Work out the finished part from the listing and answer in its coordinate system (mm). A direction names the side the tool comes from. Round coordinates to 2 decimals unless told otherwise and drop trailing zeros. Write each loop counter-clockwise with the first axis right and the second up, starting at its lowest first coordinate (ties: lowest second). Pieces come first, ordered by that corner, then holes.
1. Determine the mould class of faces 3 (the face through (1.588, 2, -7)), 4 (the face through (-5.796, 1.565, -7.559)), 5 (the face through (-2, 0, 6.2)) for opening direction X: pulls with the +X half, pulls with the -X half, needs draft (parallel to the pull), parting line crosses it, or undercut.
2. Straight lines are drawn through the part: probe 1 along X at (y, z) = (0.75, 0) (3 decimals); probe 2 along Z at (x, y) = (-5, 0.85); probe 3 along X at (y, z) = (2.4, -3.5). For each, find the intervals that lie inside material, in ascending order.
3. Flat-ended cylindrical pins translate along their axes: pin 1 Ø0.9 at (y, z) = (1, -6.5) entering from -X; pin 2 Ø1.5 at (y, z) = (0.5, 7) entering from +X; pin 3 Ø1.5 at (x, y) = (1, 2) entering from +Z. Find the tip coordinate at first contact, or state that the pin passes through.
4. Find section A-A (z = 0). Write down the section's boundary in (x, y) (3 decimals), and give its area (3 significant figures).
5. A tool of negligible diameter and unlimited length cuts with its end or side. For faces 1 (the face through (-2, 3.175, 6.2)), 2 (the face through (0, 2, -7.938)), from which of +Z, -Z, +X, -X, +Y, -Y can it reach the whole face along a straight path? Write none if from no direction.
```python
from build123d import *

# Parameters (mm, degrees)
SKETCH1_R           = 9.525
BOSS_EXTRUDE1_DEPTH = 3.175


with BuildPart() as part:
    # Sketch1 → Boss-Extrude1 (new body)
    with BuildSketch(Plane(origin=(0, 0, 0), x_dir=(1, 0, 0), z_dir=(0, 1, 0))):
        with Locations(Location((0, 0, 0), (0, 0, 270))):
            Circle(SKETCH1_R)
        with BuildLine():
            Line((-1.5875, 6.148361062), (-1.5875, 7.9375))
            Line((-1.5875, 7.9375), (1.5875, 7.9375))
            Line((1.5875, 7.9375), (1.5875, 6.148361062))
            ThreePointArc((1.5875, 6.148361062), (0, -6.35), (-1.5875, 6.148361062))
        make_face(mode=Mode.SUBTRACT)
    extrude(amount=BOSS_EXTRUDE1_DEPTH)


solid = part.part
```
Worked answers:
1. face 3: undercut
1. face 4: parting line crosses it
1. face 5: needs draft
2. probe 1: x = -9.525 to -6.35, 6.35 to 9.525
2. probe 2: z = -8.11 to -3.91, 3.91 to 8.11
2. probe 3: x = -8.86 to -5.3, 5.3 to 8.86
3. pin 1: stops at x = -7.36
3. pin 2: stops at x = 7.19
3. pin 3: stops at z = 9.52
4. outline: (-9.525, 0) - (-6.35, 0) - (-6.35, 3.175) - (-9.525, 3.175) - close; (6.35, 0) - (9.525, 0) - (9.525, 3.175) - (6.35, 3.175) - close
4. area: 20.2 mm2
5. face 1: +Z, -Z, +X, -X, +Y
5. face 2: +Y, -Y
